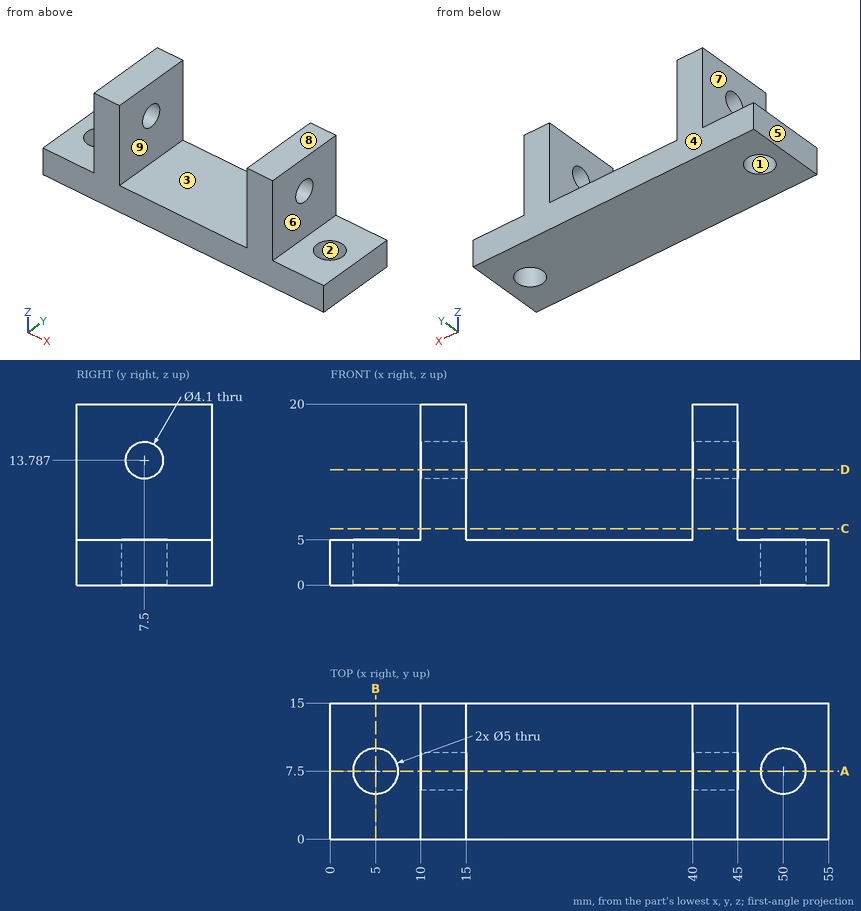
Drawing for the job (mm, zero at the part's lowest x, y, z). A direction names the side the tool comes from. Round coordinates to 2 decimals unless told otherwise and drop trailing zeros. Write each loop counter-clockwise with the first axis right and the second up, starting at its lowest first coordinate (ties: lowest second). Pieces come first, ordered by that corner, then holes. Notation, with made-up numbers: (75.25, -7.5) - (121.25, -7.5) arc R13 cw to (121.25, 4.5) - close; hole circle Ø8 at (-39, 39.25). An arc over 180 degrees is marked (long way). Use CSV: the item, a comma, the result in double quotes.
(1) Mould opens along Y. For the marked faces 1, 2, 3 and 4 say: pulls with the +Y half, pulls with the -Y half, needs draft (parallel to the pull), parting line crosses it, or undercut.
Response:
face 1,"undercut"
face 2,"undercut"
face 3,"needs draft"
face 4,"pulls with the +Y half"
(2) Wall check: line 1 (Y direction, x = 50, z = 1.5); line 2 (X direction, y = 13.25, z = 19.25); line 3 (X direction, y = 8, z = 4). Give the ranges that are in metal, low to high.
Response:
line 1,"0 to 5, 10 to 15"
line 2,"10 to 15, 40 to 45"
line 3,"0 to 2.55, 7.45 to 47.55, 52.45 to 55"
(3) Band-saw the part on A-A (y = 7.5). Write the cut outline in (x, z).
Response:
outline,"(0, 0) - (2.5, 0) - (2.5, 5) - (0, 5) - close; (7.5, 0) - (47.5, 0) - (47.5, 5) - (45, 5) - (45, 11.74) - (40, 11.74) - (40, 5) - (15, 5) - (15, 11.74) - (10, 11.74) - (10, 5) - (7.5, 5) - close; (10, 15.84) - (15, 15.84) - (15, 20) - (10, 20) - close; (40, 15.84) - (45, 15.84) - (45, 20) - (40, 20) - close; (52.5, 0) - (55, 0) - (55, 5) - (52.5, 5) - close"
(4) Band-saw the part on B-B (x = 5). Write the cut outline in (y, z), plus the area to 3 significant figures.
Response:
outline,"(0, 0) - (5, 0) - (5, 5) - (0, 5) - close; (10, 0) - (15, 0) - (15, 5) - (10, 5) - close"
area,"50.0 mm²"
(5) Pin check, flat tips, straight feed: P1, Ø6, axis at y = 3.5, z = 14.5, coming from the +X side; P2, Ø3, axis at x = 3.5, y = 5, coming from the +Z side; P3, Ø3.5, axis at y = 7.5, z = 13.79, coming from the +X side; P4, Ø4.5, axis at y = 6.5, z = 9.5, coming from the -X side. Stop position of each tip, or through.
Response:
P1,"x = 45"
P2,"z = 5"
P3,"through"
P4,"x = 10"
(6) 3-axis set-ups, long thin cutter, end or side, ignore diameter. For the marked faces 5, 6, 7, 8 and 9: which of +Z, -Z, +X, -X, +Y, -Y reach the whole face in a straight line?
Response:
face 5,"+Z, -Z, -X, +Y, -Y"
face 6,"+Z, +X, +Y, -Y"
face 7,"+Z, -X, +Y, -Y"
face 8,"+Z, +X, -X, +Y, -Y"
face 9,"+Z, +Y, -Y"
(7) Band-saw the part on C-C (z = 6.25). Write the cut outline in (x, y).
Response:
outline,"(10, 0) - (15, 0) - (15, 15) - (10, 15) - close; (40, 0) - (45, 0) - (45, 15) - (40, 15) - close"
(8) Band-saw the part on D-D (z = 12.75). Write the cut outline in (x, y), plus the area to 3 significant figures.
Response:
outline,"(10, 0) - (15, 0) - (15, 5.73) - (10, 5.73) - close; (10, 9.27) - (15, 9.27) - (15, 15) - (10, 15) - close; (40, 0) - (45, 0) - (45, 5.73) - (40, 5.73) - close; (40, 9.27) - (45, 9.27) - (45, 15) - (40, 15) - close"
area,"115 mm²"
